Could you check a few things on this model? Use its own coordinates, in mm. Coordinates: 2 decimals unless noted, no trailing zeros. Order: outer loops, then holes, each group sorted by start corner. A loop starts at its lowest first (then second) coordinate and runs counter-clockwise, first axis right, second up. Notation, with made-up numbers: M 31,-32 L 67,-32 A13 cw 67,-16 Z; hole C 23,5 d4. An arc over 180 degrees is marked long. One line per question, with ' | ' between items. Start each with the question number.
from build123d import *

# Parameters (mm, degrees)
F0_R     = 1
F1_DEPTH = 5
F2_R     = 1.5
F3_DEPTH = 1.5
F4_R     = 0.5
F5_R     = 1.5
F5_R_2   = 1
F6_DEPTH = 1.5
F7_R     = 0.5


with BuildPart() as f1:
    # F0 (on Top) → F1 (new body)
    with BuildSketch(Plane.XY):
        Circle(F0_R)
    extrude(amount=-F1_DEPTH)

    # F2 (on face) → F3 (join)
    with BuildSketch(Plane.XY):
        Circle(F2_R)
    extrude(amount=F3_DEPTH)

    # F4
    f4_edges = [f1.edges().sort_by_distance(p)[0] for p in [
        (-1.5, 0, 1.5),
    ]]
    fillet(f4_edges, radius=F4_R)

    # F5 (on face) → F6 (join)
    with BuildSketch(Plane(origin=(0, 0, -5), x_dir=(1, 0, 0), z_dir=(0, 0, -1))):
        Circle(F5_R)
        Circle(F5_R_2, mode=Mode.SUBTRACT)
        Circle(F5_R_2)
    extrude(amount=F6_DEPTH)

    # F7
    f7_edges = [f1.edges().sort_by_distance(p)[0] for p in [
        (-1.5, 0, -6.5),
    ]]
    fillet(f7_edges, radius=F7_R)


solid = f1.part
(1) Imagine slicing it at A-A, the plane y = 0. Write out the boundary of the cut face in (x, z), plus the area to 3 significant figures.
(2) We'd pull the mould along Z, two halves only. Please class faces 1 (the cylindrical face through (0, -1, -2)), 2 (the cylindrical face through (-1.5, 0.07, 0.49)), 3 (the flat face through (0, 0, 1.5)): +Z half, -Z half, draft (parallel to the pull), parting line (faces both ways), or undercut.
(3) For P1, Ø1, axis at x = 0, z = -1, coming from the -Y side, with a flat end and sliding along its axis, tell me the tip position at first contact or that it passes through.
(4) If I drill on line 1 along Z through (x, y) = (1.2, -0.6); line 2 along Y through (x, z) = (0.05, -4.5); line 3 along Z through (x, y) = (0.85, 1.1), over which ranges is the centre line in solid material (lowest first)? Write a range as from..to.
(5) Imagine slicing it at C-C, the plane z = -4. Write out the boundary of the cut face in (x, y), plus the area to 3 significant figures.
Answers:
1) outline: M -1.5,-6 A0.5 ccw -1,-6.5 L 1,-6.5 A0.5 ccw 1.5,-6 L 1.5,-5 L 1,-5 L 1,0 L 1.5,0 L 1.5,1 A0.5 ccw 1,1.5 L -1,1.5 A0.5 ccw -1.5,1 L -1.5,0 L -1,0 L -1,-5 L -1.5,-5 Z | area: 18.8 mm²
2) face 1: undercut | face 2: draft | face 3: +Z half
3) P1: y = -1
4) line 1: -6.37..-5, 0..1.37 | line 2: -1..1 | line 3: -6.31..-5, 0..1.31
5) outline: C 0,0 d2 | area: 3.14 mm²
